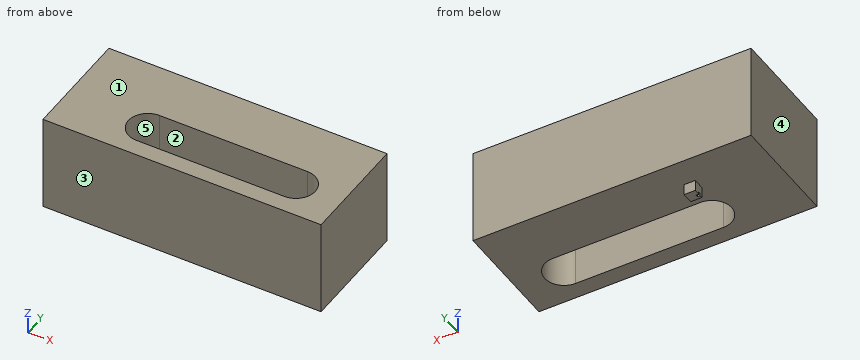
from build123d import *

# Parameters (mm, degrees)
F0_W     = 50
F0_H     = 20
F1_DEPTH = 17.5
F3_DEPTH = 50
F4_W     = 2
F4_H     = 2
F5_DEPTH = 2
F6_W     = 0.5
F6_H     = 0.45
F7_DEPTH = 0.4


with BuildPart() as f1:
    # F0 (on Top) → F1 (new body)
    with BuildSketch(Plane.XY):
        with Locations((10, 0)):
            Rectangle(F0_W, F0_H)
    extrude(amount=F1_DEPTH)

    # F2 (on Top) → F3 (cut)
    with BuildSketch(Plane.XY):
        with BuildLine():
            ThreePointArc((0, 0), (-3.5, -3.5), (0, -7))
            Line((0, -7), (26.61685, -7))
            ThreePointArc((26.61685, -7), (30.11685, -3.5), (26.61685, 0))
            Line((26.61685, 0), (0, 0))
        make_face()
    extrude(amount=F3_DEPTH, mode=Mode.SUBTRACT)

    # F4 (on face) → F5 (join)
    with BuildSketch(Plane(origin=(0, 0, 0), x_dir=(1, 0, 0), z_dir=(0, 0, -1))):
        with Locations((-1, -4)):
            Rectangle(F4_W, F4_H)
    extrude(amount=F5_DEPTH)

    # F6 (on face) → F7 (cut)
    with BuildSketch(Plane(origin=(0, 0, -2), x_dir=(1, 0, 0), z_dir=(0, 0, -1))):
        with Locations((-1.75, -3.725)):
            Rectangle(F6_W, F6_H)
    extrude(amount=-F7_DEPTH, mode=Mode.SUBTRACT)


solid = f1.part
Here's how the part is built. I have some questions about the finished solid (model axes, mm). Face numbers are marked on the shaded views. A direction names the side the tool comes from. Give positions to 0.01 mm unless a question says otherwise; leave off trailing zeros. Loops run counter-clockwise (first coordinate to the right, second up) from the corner with the lowest first, then second, coordinate; pieces in that order, holes last. Notation, with made-up numbers: (25, 27.5) -> (70, 27.5) arc R23 cw to (70, 62.5) -> close; hole circle Ø6 at (72, 19). An arc over 180 degrees is marked (long way). One line per item, written item: value.
Q1. We'd pull the mould along Y, two halves only. Please class the marked faces 1, 2 and 3: pulls with the +Y half, pulls with the -Y half, needs draft (parallel to the pull), parting line crosses it, or undercut.
Answers follow:
face 1: needs draft
face 2: undercut
face 3: pulls with the -Y half
Q2. Suppose I cut it at D-D on y = 6.25. Please give me the cut outline in (x, z), then the cut area to 3 significant figures.
Answers follow:
outline: (-15, 0) -> (35, 0) -> (35, 17.5) -> (-15, 17.5) -> close
area: 875 mm^2
Q3. I'm going to push flat-ended pins straight in: pin 1 Ø1 at (y, z) = (4, -1) entering from -X; pin 2 Ø1.5 at (x, y) = (-3.5, 7.5) entering from -Z; pin 3 Ø0.6 at (x, z) = (-1, -1.5) entering from +Y. Where does each tip first touch, or does it pass through?
Answers follow:
pin 1: x = -2
pin 2: z = 0
pin 3: y = 5
Q4. Suppose I cut it at A-A on y = -3.5. Please give me the cut outline in (x, z).
Answers follow:
outline: (-15, 0) -> (-3.5, 0) -> (-3.5, 17.5) -> (-15, 17.5) -> close; (30.12, 0) -> (35, 0) -> (35, 17.5) -> (30.12, 17.5) -> close
Q5. If I drill on line 1 along Y through (x, z) = (18.5, 4.5); line 2 along Z through (x, y) = (30, 7); line 3 along X through (y, z) = (-0.5, 14.5), over which ranges is the centre line in solid material (lowest first)?
Answers follow:
line 1: -10 to -7, 0 to 10
line 2: 0 to 17.5
line 3: -15 to -1.8, 28.42 to 35
Q6. Suppose I cut it at C-C on z = 13.75. Please give me the cut outline in (x, y).
Answers follow:
outline: (-15, -10) -> (35, -10) -> (35, 10) -> (-15, 10) -> close; hole (0, -7) -> (26.62, -7) arc R3.5 ccw to (26.62, 0) -> (0, 0) arc R3.5 ccw to start
Q7. On a 3-axis mill with a long thin cutter (end or side, diameter ignored), from which of +Z, -Z, +X, -X, +Y, -Y can I reach the whole of each face in a straight line? I mean the marked faces 4 and 5. Say none if no direction works.
Answers follow:
face 4: +Z, -Z, -X, +Y, -Y
face 5: +Z, -Z
Q8. Suppose I cut it at B-B on x = 10.5. Please give me the cut outline in (y, z), then the cut area to 4 significant figures.
Answers follow:
outline: (-10, 0) -> (-7, 0) -> (-7, 17.5) -> (-10, 17.5) -> close; (0, 0) -> (10, 0) -> (10, 17.5) -> (0, 17.5) -> close
area: 227.5 mm^2
